from build123d import *

# Parameters (mm, degrees)
SKETCH_1_W      = 32
SKETCH_1_H      = 14
SKETCH_1_W_2    = 74
SKETCH_1_H_2    = 64
SKETCH_1_R      = 1.6
SKETCH_1_W_3    = 14
SKETCH_1_H_3    = 32
EXTRUDE_1_DEPTH = 2
CHAMFER_1_SIZE  = 1.4
SKETCH_2_W      = 10.4
SKETCH_2_H      = 43.2
SKETCH_2_W_2    = 102.4
SKETCH_2_H_2    = 10.4
SKETCH_2_W_3    = 70.4
SKETCH_2_H_3    = 10
SKETCH_2_H_4    = 11.2
EXTRUDE_2_DEPTH = 2
FILLET_1_R      = 1.8


with BuildPart() as part:
    # 草图1 → 凸台-拉伸1 (new body)
    # profile 1 of 5: a face of its own
    with BuildSketch(Plane.XY):
        with Locations((-34, 12)):
            Rectangle(SKETCH_1_W, SKETCH_1_H)
    # profile 2 of 5: a face of its own
    with BuildSketch(Plane.XY):
        with Locations((-34, 36)):
            Rectangle(SKETCH_1_W, SKETCH_1_H)
    # profile 3 of 5: a face of its own
    with BuildSketch(Plane.XY):
        with Locations((19, 24)):
            Rectangle(SKETCH_1_W_2, SKETCH_1_H_2)
        with Locations((0, 48)):
            Circle(SKETCH_1_R, mode=Mode.SUBTRACT)
        with Locations((0, 24)):
            Circle(SKETCH_1_R, mode=Mode.SUBTRACT)
        with Locations((38, 48)):
            Circle(SKETCH_1_R, mode=Mode.SUBTRACT)
        with Locations((38, 24)):
            Circle(SKETCH_1_R, mode=Mode.SUBTRACT)
        with Locations((38, 0)):
            Circle(SKETCH_1_R, mode=Mode.SUBTRACT)
        Circle(SKETCH_1_R, mode=Mode.SUBTRACT)
    # profile 4 of 5: a face of its own
    with BuildSketch(Plane.XY):
        with Locations((-11, -24)):
            Rectangle(SKETCH_1_W_3, SKETCH_1_H_3)
    # profile 5 of 5: a face of its own
    with BuildSketch(Plane.XY):
        with Locations((49, -24)):
            Rectangle(SKETCH_1_W_3, SKETCH_1_H_3)
    extrude(amount=EXTRUDE_1_DEPTH)

    # 倒角1
    chamfer_1_edges = [part.edges().sort_by_distance(p)[0] for p in [
        (-1.6, 0, 0),
        (36.4, 0, 0),
        (36.4, 24, 0),
        (36.4, 48, 0),
        (-1.6, 24, 0),
        (-1.6, 48, 0),
    ]]
    chamfer(chamfer_1_edges, length=CHAMFER_1_SIZE)

    # 草图2 → 凸台-拉伸2 (add)
    with BuildSketch(Plane(origin=(0, 0, 0), x_dir=(-1, 0, 0), z_dir=(0, 0, -1))):
        Polygon((-56, 56), (-56, -40), (-42, -40), (-42, 5), (4, 5), (4, -40), (18, -40), (18, 5), (50, 5), (50, 19), (18, 19), (18, 29), (50, 29), (50, 43), (18, 43), (18, 56), align=None)
        with Locations((11, -16.6)):
            Rectangle(SKETCH_2_W, SKETCH_2_H, mode=Mode.SUBTRACT)
        with Locations((-49, -16.6)):
            Rectangle(SKETCH_2_W, SKETCH_2_H, mode=Mode.SUBTRACT)
        with Locations((-3, 12)):
            Rectangle(SKETCH_2_W_2, SKETCH_2_H_2, mode=Mode.SUBTRACT)
        with Locations((-19, 24)):
            Rectangle(SKETCH_2_W_3, SKETCH_2_H_3, mode=Mode.SUBTRACT)
        with Locations((-3, 36)):
            Rectangle(SKETCH_2_W_2, SKETCH_2_H_2, mode=Mode.SUBTRACT)
        with Locations((-19, 48.6)):
            Rectangle(SKETCH_2_W_3, SKETCH_2_H_4, mode=Mode.SUBTRACT)
    extrude(amount=EXTRUDE_2_DEPTH)

    # 圆角1
    fillet_1_edges = [part.edges().sort_by_distance(p)[0] for p in [
        (-18, 19, 0),
        (-18, 29, 0),
        (-50, 29, 0),
        (-50, 43, 0),
        (-18, 43, 0),
        (-18, 56, 0),
        (56, 56, 0),
        (42, -40, 0),
        (42, -8, 1),
        (-4, -8, 1),
        (-4, -40, 0),
        (-18, -40, 0),
        (-18, 5, 0),
        (-50, 5, 0),
        (-50, 19, 0),
    ]]
    fillet(fillet_1_edges, radius=FILLET_1_R)


solid = part.part
Geometry: final body of the model. Coordinates: model frame, mm. A direction names the side the tool comes from. Coordinates: 2 decimals unless noted, no trailing zeros. Loops run counter-clockwise (first coordinate to the right, second up) from the corner with the lowest first, then second, coordinate; pieces in that order, holes last. Notation, with made-up numbers: (33.5, 54) - (86.5, 54) arc R16 cw to (86.5, 68) - close; hole circle Ø1 at (6.25, -32.5). An arc over 180 degrees is marked (long way). Put each result on its own line as item: value. Start each with the question number.
Q1. Pull-direction query (X, two-part tool) for faces 1 (the flat face through (19, 56, 0)), 2 (the flat face through (-50, 12, 0)), 3 (the flat face through (49, -16, 0)), 4 (the flat face through (2, 36, 0)); classes: released by +X, released by -X, zero draft, split by the parting line, or undercut.
Q2. Cut plane D-D, the plane x = 26. Return loops of the section in (y, z).
Q3. Pin query (flat end, axial travel): pin 1 Ø2 at (y, z) = (51.5, -0.5) entering from -X; pin 2 Ø5 at (x, y) = (-18.5, 13) entering from -Z; pin 3 Ø1.6 at (x, z) = (25, -1.5) entering from -Y; pin 4 Ø1.5 at (x, y) = (37.5, 0.5) entering from +Z. Return the tip coordinate at first contact, or that it passes through.
Q4. Cut plane B-B, the plane y = -18. Return loops of the section in (x, z).
Q5. Set-up query: faces 5 (the flat face through (-34, 5, 0)), 6 (the flat face through (-18, 49, 0)), 7 (the flat face through (2, 12, 0)), 8 (the cylindrical face through (36.82, 1.08, 1.7)). Return all of +Z, -Z, +X, -X, +Y, -Y with unobstructed straight access to the full face (end or side cutting, diameter ignored); none if empty.
Q6. Cut plane C-C, the plane x = -23.5. Return loops of the section in (y, z).
Q7. Cut plane A-A, the plane y = 48. Return loops of the section in (x, z), and give its area (3 significant figures).
Q8. Line query: line 1 (Y direction, x = 0, z = 1.7); line 2 (X direction, y = -32, z = -0.3); line 3 (Y direction, x = 33, z = -0.6). Output: solid intervals per line, ascending.
Filled sheet:
1. face 1: zero draft
1. face 2: released by -X
1. face 3: undercut
1. face 4: undercut
2. outline: (-8, 0) - (5, 0) - (5, -2) - (6.8, -2) - (6.8, 0) - (17.2, 0) - (17.2, -2) - (19, -2) - (19, 0) - (29, 0) - (29, -2) - (30.8, -2) - (30.8, 0) - (41.2, 0) - (41.2, -2) - (43, -2) - (43, 0) - (54.2, 0) - (54.2, -2) - (56, -2) - (56, 2) - (-8, 2) - close
3. pin 1: x = -18
3. pin 2: z = 0
3. pin 3: y = 5
3. pin 4: through
4. outline: (-18, -2) - (-16.2, -2) - (-16.2, 0) - (-5.8, 0) - (-5.8, -2) - (-4, -2) - (-4, 2) - (-18, 2) - close; (42, -2) - (43.8, -2) - (43.8, 0) - (54.2, 0) - (54.2, -2) - (56, -2) - (56, 2) - (42, 2) - close
5. face 5: +Z, -Z, -X, -Y
5. face 6: +Z, -Z, -X, +Y
5. face 7: -Z
5. face 8: +Z, -Z
6. outline: (5, -2) - (6.8, -2) - (6.8, 0) - (17.2, 0) - (17.2, -2) - (19, -2) - (19, 2) - (5, 2) - close; (29, -2) - (30.8, -2) - (30.8, 0) - (41.2, 0) - (41.2, -2) - (43, -2) - (43, 2) - (29, 2) - close
7. outline: (-18, -2) - (-16.2, -2) - (-16.2, 0) - (-3, 0) - (-1.6, 1.4) - (-1.6, 2) - (-18, 2) - close; (1.6, 1.4) - (3, 0) - (35, 0) - (36.4, 1.4) - (36.4, 2) - (1.6, 2) - close; (39.6, 1.4) - (41, 0) - (54.2, 0) - (54.2, -2) - (56, -2) - (56, 2) - (39.6, 2) - close
7. area: 138 mm²
8. line 1: -8 to -1.6, 1.6 to 22.4, 25.6 to 46.4, 49.6 to 56
8. line 2: -18 to -16.2, -5.8 to -4, 42 to 43.8, 54.2 to 56
8. line 3: 5 to 6.8, 17.2 to 19, 29 to 30.8, 41.2 to 43, 54.2 to 56
